Design review of the part shown in the three views and the two pictorial views. Dimensions are in mm from the part's minimum x, y and z. A direction names the side the tool comes from. Round coordinates to 2 decimals unless told otherwise and drop trailing zeros. Loops run counter-clockwise (first coordinate to the right, second up) from the corner with the lowest first, then second, coordinate; pieces in that order, holes last. Notation, with made-up numbers: M 83,84.25 L 106,84.25 A16 cw 106,98.25 Z; hole C 72.25,84 d3. An arc over 180 degrees is marked long. One line per question, with ' | ' between items.
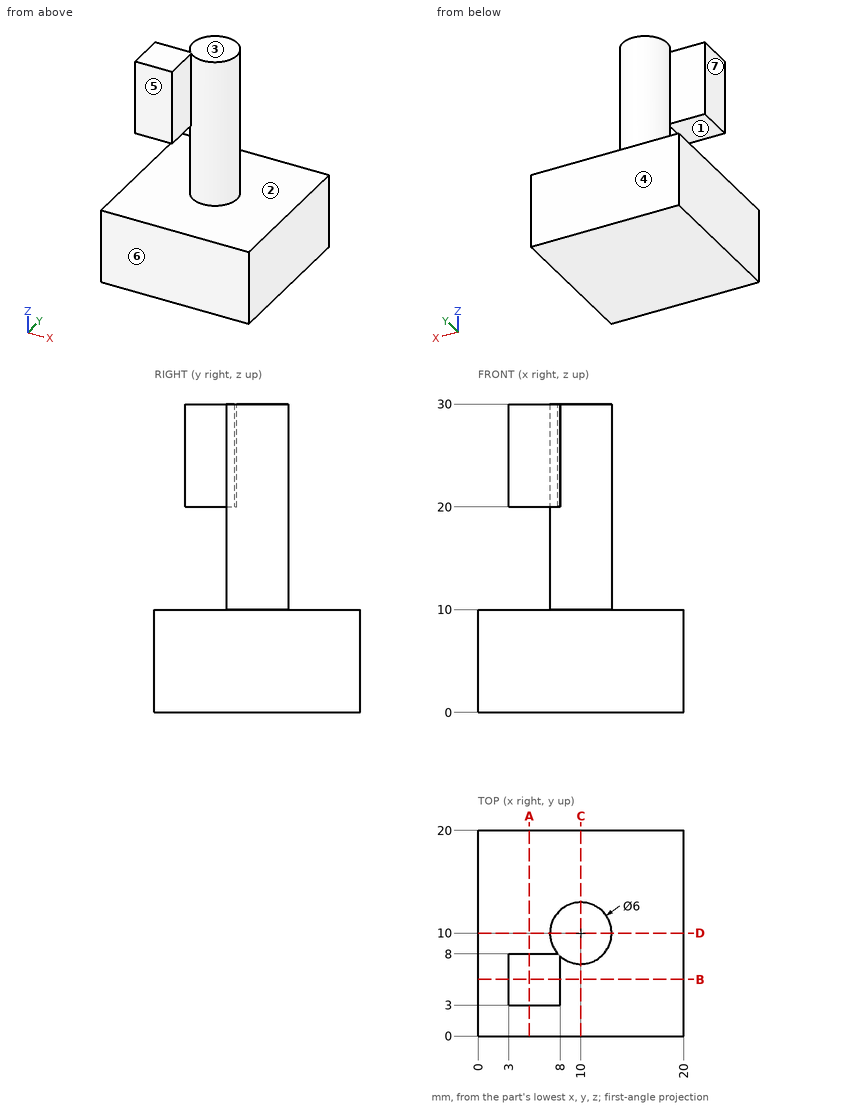
1) Mouldability with a two-part tool opening along Z and no side actions: class the marked faces 1, 2, 3 and 4 as +Z half, -Z half, draft (parallel to the pull), parting line (faces both ways), or undercut.
Output values:
face 1: undercut | face 2: undercut | face 3: +Z half | face 4: draft
2) Insertion check: P1, Ø6, axis at x = 7, z = 22, coming from the -Y side; P2, Ø2.5, axis at y = 4.5, z = 22.5, coming from the -X side; P3, Ø12, axis at y = 17, z = 23, coming from the +X side; P4, Ø3, axis at y = 4, z = 15, coming from the -X side. Each pin has a flat end and moves straight along its axis. Give the tip position at first contact, or say it passes through.
Output values:
P1: stops at y = 3 | P2: stops at x = 3 | P3: stops at x = 12.83 | P4: passes through
3) Add section C-C on x = 10. State the section outline as (y, z) points, then the cut area to 3 significant figures.
Output values:
outline: M 0,0 L 20,0 L 20,10 L 13,10 L 13,30 L 7,30 L 7,10 L 0,10 Z | area: 320 mm²
4) For line 1 (Y direction, x = 4, z = 24.5); line 2 (Z direction, x = 8, y = 14.5); line 3 (Y direction, x = 10, z = 11.75), list the stretches that pass through material, from the lowest coordinate up.
Output values:
line 1: y = 3 to 8 | line 2: z = 0 to 10 | line 3: y = 7 to 13
5) Machinability: for the marked faces 5, 6 and 7, which of the approach directions +Z, -Z, +X, -X, +Y, -Y give a long, thin tool a straight path to every point of the face, cutting with its end or side? Answer none if there is none.
Output values:
face 5: +Z, +X, -X, -Y | face 6: +Z, -Z, +X, -X, -Y | face 7: +Z, -X, +Y, -Y
6) Add section A-A on x = 5. State the section outline as (y, z) points, then the cut area to 3 significant figures.
Output values:
outline: M 0,0 L 20,0 L 20,10 L 0,10 Z; M 3,20 L 8,20 L 8,30 L 3,30 Z | area: 250 mm²
